```python
from build123d import *

# Parameters (mm, degrees)
SKETCH_1_W      = 28.6
SKETCH_1_H      = 15.3
EXTRUDE_1_DEPTH = 1
SKETCH_2_W      = 4.6
SKETCH_2_H      = 9.6
EXTRUDE_2_DEPTH = 2.5
SKETCH_3_W      = 0.4
SKETCH_3_H      = 0.4
EXTRUDE_3_DEPTH = 5.6


with BuildPart() as part:
    # 草图1 → 凸台-拉伸1 (new body)
    with BuildSketch(Plane(origin=(0, 0, 0), x_dir=(1, 0, 0), z_dir=(0, 1, 0))):
        Rectangle(SKETCH_1_W, SKETCH_1_H)
    extrude(amount=EXTRUDE_1_DEPTH)

    # 草图2 → 凸台-拉伸2 (add)
    with BuildSketch(Plane.XZ):
        with Locations((11.5, 2.05)):
            Rectangle(SKETCH_2_W, SKETCH_2_H)
    extrude(amount=EXTRUDE_2_DEPTH)

    # 草图3 → 凸台-拉伸3 (add)
    with BuildSketch(Plane.XZ.offset(2.5)):
        with Locations((12.75, 5.65)):
            Rectangle(SKETCH_3_W, SKETCH_3_H)
        with Locations((10.35, 5.65)):
            Rectangle(SKETCH_3_W, SKETCH_3_H)
        with Locations((12.75, 3.25)):
            Rectangle(SKETCH_3_W, SKETCH_3_H)
        with Locations((12.75, 0.85)):
            Rectangle(SKETCH_3_W, SKETCH_3_H)
        with Locations((12.75, -1.55)):
            Rectangle(SKETCH_3_W, SKETCH_3_H)
        with Locations((10.35, 3.25)):
            Rectangle(SKETCH_3_W, SKETCH_3_H)
        with Locations((10.35, 0.85)):
            Rectangle(SKETCH_3_W, SKETCH_3_H)
        with Locations((10.35, -1.55)):
            Rectangle(SKETCH_3_W, SKETCH_3_H)
    extrude(amount=EXTRUDE_3_DEPTH)


solid = part.part
```
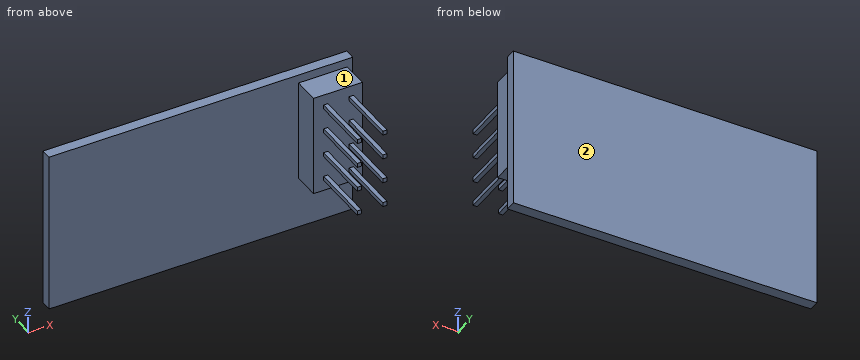
Check sheet for the modelled part. Datum: model origin and axes. Units: mm. Face numbers are marked on the shaded views. A direction names the side the tool comes from. Coordinates: 2 decimals unless noted, no trailing zeros. Order: outer loops, then holes, each group sorted by start corner. A loop starts at its lowest first (then second) coordinate and runs counter-clockwise, first axis right, second up. Notation, with made-up numbers: (5.5, 87.25) -> (24.5, 87.25) arc R31 ccw to (24.5, 126.25) -> close; hole circle Ø6 at (18, 7.25). An arc over 180 degrees is marked (long way). Write each question's results on one line, items separated by ' | '. Start each with the question number.
1) Depth check by flat-ended pin: pin 1 (1 mm diameter, centred on y = -2.5, z = -3, fed in from -X); pin 2 (1.5 mm diameter, centred on x = 3.5, z = -5.5, fed in from -Y); pin 3 (3 mm diameter, centred on y = -4.5, z = 5.5, fed in from -X). Enter the tip coordinate at first touch or a pass-through.
2) Material ranges on line 1 along X through (y, z) = (-5.5, 1); line 2 along Y through (x, z) = (11, -5.25); line 3 along X through (y, z) = (-0.5, 1), recorded low to high.
3) Section check C-C (x = -1.5). Enter the section's corners in (y, z).
4) Section check D-D (y = -2). Enter the section's corners in (x, z), and give its area (3 significant figures).
5) Set-up check for the marked faces 1 and 2: record each of +Z, -Z, +X, -X, +Y, -Y from which the full face is reachable in a straight line by a thin tool's end or side.
6) Section check A-A (y = -3.75). Count the separate pieces of the cut face and the enclosed holes in it, and give its area (3 significant figures).
7) Section check B-B (z = 0.25). Enter the section's corners in (x, y), and give its area (3 significant figures).
Checked values:
1) pin 1: x = 9.2 | pin 2: y = 0 | pin 3: x = 10.15
2) line 1: 10.15 to 10.55, 12.55 to 12.95 | line 2: 0 to 1 | line 3: 9.2 to 13.8
3) outline: (0, -7.65) -> (1, -7.65) -> (1, 7.65) -> (0, 7.65) -> close
4) outline: (9.2, -2.75) -> (13.8, -2.75) -> (13.8, 6.85) -> (9.2, 6.85) -> close | area: 44.2 mm²
5) face 1: +Z, +X, -X, -Y | face 2: +Z, -Z, +X, -X, +Y
6) separate pieces: 8 | enclosed holes: 0 | area: 1.28 mm²
7) outline: (-14.3, 0) -> (9.2, 0) -> (9.2, -2.5) -> (13.8, -2.5) -> (13.8, 0) -> (14.3, 0) -> (14.3, 1) -> (-14.3, 1) -> close | area: 40.1 mm²
